Autodesk Inventor part; units mm, degrees
ref_plane "YZ Plane" through (0, 0, 0) normal (1, 0, 0) x (0, 1, 0)
ref_plane "XZ Plane" through (0, 0, 0) normal (0, 1, 0) x (-1, 0, 0)
ref_plane "XY Plane" through (0, 0, 0) normal (0, 0, 1) x (1, 0, 0)
sketch "スケッチ1" plane through (0, 0, 0) normal (0, 0, 1) x (1, 0, 0)
  line L0 (-50, 0) -> (50, 0) construction
  circle A0 centre (-50, 0) radius 4.05
  circle A1 centre (50, 0) radius 4.05
  line L1 (-50, 8.5) -> (43, 8.5)
  line L2 (-50, -8.5) -> (43, -8.5)
  arc A2 (-50, 8.5) -> (-50, -8.5) centre (-50, 0) ccw
  arc A3 (25.013, -3.45) -> (25.013, 3.45) centre (25.013, 0) ccw
  line L3 (25.013, -3.45) -> (-2, -3.45)
  line L4 (25.013, 3.45) -> (-2, 3.45)
  arc A4 (-2, 3.45) -> (-2, -3.45) centre (-2, 0) ccw
  line L5 (43, -8.5) -> (50.0601, -8.4498)
  line L6 (43, 8.5) -> (50.0601, 8.4498)
  arc A5 (50.0601, -8.4498) -> (50.0601, 8.4498) centre (50, 0) ccw
  line L7 (-41, -8.5) -> (-12, -8.5) construction
  line L8 (-12, -8.5) -> (-12, -3.5) construction
  line L9 (-12, -3.5) -> (-41, -3.5) construction
  line L10 (-41, -3.5) -> (-41, -8.5) construction
  line L11 (-41, -6) -> (-12, -6) construction
  circle A6 centre (-26.5, -6) radius 1.55
  circle A7 centre (-38.5, -6) radius 1.55
  circle A8 centre (-14.5, -6) radius 1.55
  line L12 (-26.5, -6) -> (-26.5, -3.5) construction
  line L13 (0, 13) -> (-30, 13)
  line L14 (-30, 13) -> (-40, 8.5)
  line L15 (0, 13) -> (10, 8.5)
  point P0 (0, 0)
  point P1 (0, 0)
  dimension "d0" = 100
  dimension "d1" = 8.1
  dimension "d2" = 8.5
  dimension "d5" = 3.45
  dimension "d7" = 52
  dimension "d8" = 8.1
  dimension "d9" = 7
  dimension "d10" = 8.45
  dimension "d11" = 27.013
  dimension "d12" = 5
  dimension "d13" = 29
  dimension "d14" = 3.1
  dimension "d15" = 2.5
  dimension "d16" = 9
  dimension "d17" = 13
  dimension "d19" = 10
  dimension "d20" = 30
  dimension "d22" = 10
  dimension "d23" = 40
  dimension "d24" = 0
extrude "押し出し1" add sketch "スケッチ1" along normal blind 2
fillet "フィレット1" radius 2 4 edges at (-40, 8.5, 1) (-30, 13, 1) (0, 13, 1) (43, 8.5, 1)
sketch "スケッチ2" plane through (0, 0, 0) normal (0, 0, -1) x (-1, 0, 0)
  circle A0 centre (38.5, -6) radius 1.55
  circle A1 centre (38.5, -6) radius 1.55
  circle A2 centre (26.5, -6) radius 1.55
  circle A3 centre (26.5, -6) radius 1.55
  circle A4 centre (14.5, -6) radius 1.55
  circle A5 centre (14.5, -6) radius 1.55
  point P0 (0, 0)
extrude "押し出し2" add sketch "スケッチ2" against normal up to surface (2 mm away)
equation "\"d7\" = 2 * d28"
equation "\"d8\" = d1"
equation "\"d11\" = d39"
equation "\"d19\" = d18"
equation "\"d22\" = d19"
properties part number "rinnku" material "GFRP"
Check sheet for the modelled part. Datum: model origin and axes. Units: mm. A direction names the side the tool comes from. Coordinates: 2 decimals unless noted, no trailing zeros. Write each loop counter-clockwise with the first axis right and the second up, starting at its lowest first coordinate (ties: lowest second). Pieces come first, ordered by that corner, then holes. Notation, with made-up numbers: M -13.5,72 L 0.5,72 A19 ccw 0.5,82 Z; hole C 50,82 d3. An arc over 180 degrees is marked long. Write item = value, one per line. Start each with the question number.
1. Sectioned sample at B-B (y = 0). Record the cut outline in (x, z), then the cut area to 3 significant figures.
2. Mould release check, pull along X, two halves, no side actions. Record for faces 5 (the cylindrical face through (-5.45, -0.08, 0.99)), 6 (the flat face through (-1, 5, 2)), 7 (the cylindrical face through (58.45, 0.18, 0.99)): pulls with the +X half, pulls with the -X half, needs draft (parallel to the pull), parting line crosses it, or undercut.
3. Tool access check on faces 1 (the flat face through (-1, 5, 0)), 2 (the flat face through (-45, 8.5, 1)), 3 (the flat face through (26, 8.5, 1)), 4 (the flat face through (12, -3.45, 1)). Record the directions out of +Z, -Z, +X, -X, +Y, -Y that give a thin tool (end or side, any length) a straight path to the whole face; none if there is none.
4. Sectioned sample at D-D (x = -36.5). Record the cut outline in (y, z) (3 decimals), then the cut area to 4 significant figures.
5. Go/stop test with flat-tipped pins: pin 1 (0.6 mm diameter, centred on x = 24.5, z = 0.5, fed in from +Y); pin 2 (6.5 mm diameter, centred on x = 50, y = 0, fed in from +Z); pin 3 (0.6 mm diameter, centred on x = 9, z = 0.5, fed in from +Y) (3 decimals). Record where each tip stops, or that it passes through.
6. Thickness scan on probe 1 along Y at (x, z) = (17.5, 0.6); probe 2 along Y at (x, z) = (-50, 0.4); probe 3 along Y at (x, z) = (31.5, 1.5). Record the ranges inside material, lowest first.
7. Sectioned sample at A-A (z = 1.25). Record the cut outline in (x, y).
8. Sectioned sample at C-C (x = 48). Record the cut outline in (y, z), then the cut area to 3 significant figures.
The answers:
q1.outline = M -58.5,0 L -54.05,0 L -54.05,2 L -58.5,2 Z; M -45.95,0 L -5.45,0 L -5.45,2 L -45.95,2 Z; M 28.46,0 L 45.95,0 L 45.95,2 L 28.46,2 Z; M 54.05,0 L 58.45,0 L 58.45,2 L 54.05,2 Z
q1.area = 134 mm²
q2.face_5 = undercut
q2.face_6 = needs draft
q2.face_7 = pulls with the +X half
q3.face_1 = -Z, +X, -X, +Y, -Y
q3.face_2 = +Z, -Z, -X, +Y
q3.face_3 = +Z, -Z, +X, +Y
q3.face_4 = +Z, -Z
q4.outline = M -8.5,0 L 10.075,0 L 10.075,2 L -8.5,2 Z
q4.area = 37.15 mm²
q5.pin_1 = 8.5
q5.pin_2 = through
q5.pin_3 = 9.085
q6.probe_1 = -8.5 to -3.45, 3.45 to 8.5
q6.probe_2 = -8.5 to -4.05, 4.05 to 8.5
q6.probe_3 = -8.5 to 8.5
q7.outline = M -50,-8.5 L 43,-8.5 L 50.06,-8.45 A8.45 ccw 50.06,8.45 L 43,8.5 L 10,8.5 L 0.39,12.82 A2 ccw -0.43,13 L -29.57,13 A2 ccw -30.39,12.82 L -39.61,8.68 A2 cw -40.43,8.5 L -50,8.5 A8.5 ccw Z; hole C -50,0 d8.1; hole M -2,-3.45 L 25.01,-3.45 A3.45 ccw 25.01,3.45 L -2,3.45 A3.45 ccw Z; hole C 50,0 d8.1
q8.outline = M -8.46,0 L -3.52,0 L -3.52,2 L -8.46,2 Z; M 3.52,0 L 8.46,0 L 8.46,2 L 3.52,2 Z
q8.area = 19.8 mm²
